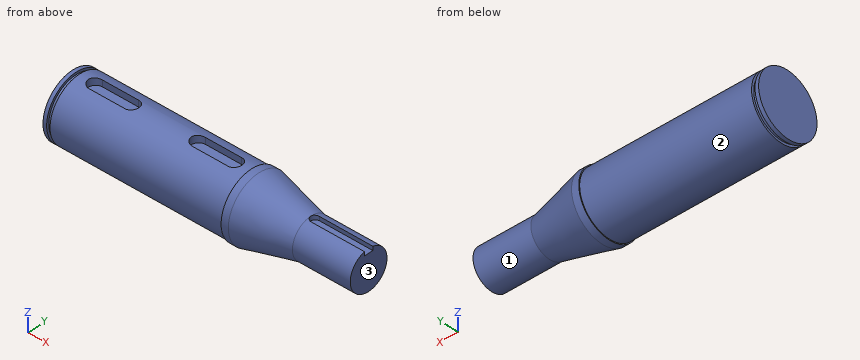
```python
from build123d import *

# Parameters (mm, degrees)
F5_DEPTH = 6.35
F7_DEPTH = 3.96875


with BuildPart() as f1:
    # F0 (on Front) → F1 (revolve)
    with BuildSketch(Plane.XZ):
        Polygon((-157.1752, 27.7495), (-157.1752, 0), (103.1748, 0), (103.1748, 17.4625), (52.3748, 17.4625), (6.35, 28.575), (0, 28.575), (0, 27.7495), (-150.9903, 27.7495), (-150.9903, 25.6794), (-153.9875, 25.6794), (-153.9875, 27.7495), align=None)
    revolve(axis=Axis((-27.0002, 0, 0), (1, 0, 0)))

    # F4 (on offset) → F5 (cut)
    with BuildSketch(Plane.XY.offset(27.7495)):
        with BuildLine():
            Line((-104.7877, 6.35), (-136.5377, 6.35))
            ThreePointArc((-136.5377, 6.35), (-142.8877, 0), (-136.5377, -6.35))
            Line((-136.5377, -6.35), (-104.7877, -6.35))
            ThreePointArc((-104.7877, -6.35), (-98.4377, 0), (-104.7877, 6.35))
        make_face()
        with BuildLine():
            Line((-14.3002, 6.35), (-46.0502, 6.35))
            ThreePointArc((-46.0502, 6.35), (-52.4002, 0), (-46.0502, -6.35))
            Line((-46.0502, -6.35), (-14.3002, -6.35))
            ThreePointArc((-14.3002, -6.35), (-7.9502, 0), (-14.3002, 6.35))
        make_face()
    extrude(amount=-F5_DEPTH, mode=Mode.SUBTRACT)

    # F6 (on offset) → F7 (cut)
    with BuildSketch(Plane.XY.offset(17.4625)):
        with BuildLine():
            Line((103.1748, 3.96875), (56.34355, 3.96875))
            ThreePointArc((56.34355, 3.96875), (52.3748, 0), (56.34355, -3.96875))
            Line((56.34355, -3.96875), (103.1748, -3.96875))
            Line((103.1748, -3.96875), (103.1748, 3.96875))
        make_face()
    extrude(amount=-F7_DEPTH, mode=Mode.SUBTRACT)


solid = f1.part
```
Input: part model. Units: mm. Frame: model coordinates. Face numbers are marked on the shaded views. A direction names the side the tool comes from. Coordinates: 2 decimals unless noted, no trailing zeros. Write each loop counter-clockwise with the first axis right and the second up, starting at its lowest first coordinate (ties: lowest second). Pieces come first, ordered by that corner, then holes.
1) Material intervals for line 1 along Y through (x, z) = (-75.5, -10.5); line 2 along Z through (x, y) = (-52, 0.5) (1 decimal); line 3 along Y through (x, z) = (-129, 25), sorted ascending.
2) Set-up query: the marked faces 1, 2 and 3. Return all of +Z, -Z, +X, -X, +Y, -Y with unobstructed straight access to the full face (end or side cutting, diameter ignored); none if empty.
3) Section C-C on x = -75. Output: boundary loops of the cut face in (y, z).
4) Section B-B on x = 73. Output: boundary loops of the cut face in (y, z) (1 decimal).
5) Section D-D on x = -114. Output: boundary loops of the cut face in (y, z).
6) Pin query (flat end, axial travel): pin 1 Ø8 at (y, z) = (-17.5, 22) entering from -X; pin 2 Ø4 at (x, z) = (90, 16) entering from -Y; pin 3 Ø3 at (x, z) = (-30.5, 25.5) entering from +Y; pin 4 Ø4 at (x, z) = (-125, -5) entering from -Y. Return the tip coordinate at first contact, or that it passes through.
Check result:
1. line 1: y = -25.69 to 25.69
1. line 2: z = -27.7 to 21.4
1. line 3: y = -12.04 to -6.35, 6.35 to 12.04
2. face 1: +X
2. face 2: -X
2. face 3: +Z, -Z, +X, +Y, -Y
3. outline: circle Ø55.5 at (0, 0)
4. outline: (-4, 13.5) - (-4, 17) arc R17.5 ccw (long way) to (4, 17) - (4, 13.5) - close
5. outline: (-6.35, 21.4) - (-6.35, 27.01) arc R27.75 ccw (long way) to (6.35, 27.01) - (6.35, 21.4) - close
6. pin 1: stops at x = -157.18
6. pin 2: stops at y = -10.44
6. pin 3: stops at y = 13.93
6. pin 4: stops at y = -27.59
